Input: part model. Units: mm. Frame: model coordinates. A direction names the side the tool comes from. Coordinates: 2 decimals unless noted, no trailing zeros. Loops run counter-clockwise (first coordinate to the right, second up) from the corner with the lowest first, then second, coordinate; pieces in that order, holes last.
```python
from build123d import *

# Parameters (mm, degrees)
F2_R     = 3.75
F3_DEPTH = 33


with BuildPart() as f1:
    # F0 (on Right) → F1 (revolve)
    with BuildSketch(Plane.YZ):
        with BuildLine():
            Line((38, 45), (8, 45))
            Line((8, 45), (8, 39))
            Line((8, 39), (0, 39))
            Line((0, 39), (0, 31))
            Line((0, 31), (30, 29))
            Line((30, 29), (30, 26))
            Line((30, 26), (72, 26))
            Line((72, 26), (72, 0))
            Line((72, 0), (90, 0))
            Line((90, 0), (90, 32))
            Line((90, 32), (93, 32))
            Line((93, 32), (93, 39))
            Line((93, 39), (60, 39))
            Line((60, 39), (45.8678821818, 29.1045845728))
            ThreePointArc((45.8678821818, 29.1045845728), (40.6912569338, 28.7652906284), (38, 33.2003447942))
            Line((38, 33.2003447942), (38, 45))
        make_face()
    revolve(axis=Axis((0, 81, 0), (0, -1, 0)))

    # F2 (on face) → F3 (join)
    with BuildSketch(Plane(origin=(0, 93, 0), x_dir=(-1, 0, 0), z_dir=(0, 1, 0))):
        with BuildLine():
            Line((-8.2742985586, 74.4249113641), (-34.130188626, 18.8714128871))
            ThreePointArc((-34.130188626, 18.8714128871), (1.513291562, 38.9706293078), (35.4908216229, 16.1679182498))
            Line((35.4908216229, 16.1679182498), (8.9837408504, 74.3546347403))
            ThreePointArc((8.9837408504, 74.3546347403), (0.3772254297, 79.9162169156), (-8.2742985586, 74.4249113641))
        make_face()
        with Locations((0.3385407115, 70.4162956794)):
            Circle(F2_R, mode=Mode.SUBTRACT)
        with BuildLine():
            Line((-35.0538594373, -17.094646488), (-8.4168125088, -71.7159163408))
            ThreePointArc((-8.4168125088, -71.7159163408), (0.1390979946, -77.0518203061), (8.6756874862, -71.6850600617))
            Line((8.6756874862, -71.6850600617), (35.1153510684, -16.9679733422))
            ThreePointArc((35.1153510684, -16.9679733422), (0.0704047345, -38.9999364509), (-35.0538594373, -17.094646488))
        make_face()
        with Locations((0.1219481234, -67.551835786)):
            Circle(F2_R, mode=Mode.SUBTRACT)
    extrude(amount=-F3_DEPTH)


solid = f1.part
```
Item 1: Line query: L1, parallel to Z at x = 0, y = 91.3; L2, parallel to X at y = 61, z = 0; L3, parallel to Y at x = -38.5, z = -14. Output: solid intervals per line, ascending.
Result:
L1: z = -77.05 to -71.3, -63.8 to -32, 32 to 66.68, 74.15 to 79.91
L2: x = -39 to -26, 26 to 39
L3: y = 8 to 38
Item 2: Reachability of faces 4 (the face through (21.02, 76.73, 47.04)), 5 (the face through (-37, 8, -14)), 6 (the face through (21.922, 76.731, -44.023)), 7 (the face through (-22.4, 76.7, 44.9)), 8 (the face through (30, 38, 17)) from +Z, -Z, +X, -X, +Y, -Y: full face, straight path, thin tool, end or side. Return the list, or none.
Result:
face 4: +Z, +X, +Y
face 5: -Y
face 6: -Z, +X, +Y
face 7: +Z, -X, +Y
face 8: none
Item 3: Section query A-A (y = 78). Output: boundary loops of the cut face in (x, z), then the cut area to 3 significant figures.
Result:
outline: (-35.49, 16.17) arc R39 ccw to (-35.12, -16.97) - (-8.68, -71.69) arc R9.5 ccw to (8.42, -71.72) - (35.05, -17.09) arc R39 ccw to (34.13, 18.87) - (8.27, 74.42) arc R9.5 ccw to (-8.98, 74.35) - close; hole circle Ø7.5 at (-0.34, 70.42); hole circle Ø7.5 at (-0.12, -67.55)
area: 7,510 mm2
Item 4: Section query D-D (y = 16). Output: boundary loops of the cut face in (x, z).
Result:
outline: circle Ø90 at (0, 0); hole circle Ø59.87 at (0, 0)
Item 5: Section query B-B (x = 0). Count the separate pieces of the cut face and the enclosed holes in it, then the cut area to 3 significant figures.
Result:
separate pieces: 3
enclosed holes: 0
area: 5,250 mm2
Item 6: Section query C-C (z = 0). Output: boundary loops of the cut face in (x, y), then the cut area to 3 significant figures.
Result:
outline: (-45, 8) - (-39, 8) - (-39, 0) - (-31, 0) - (-29, 30) - (-26, 30) - (-26, 72) - (26, 72) - (26, 30) - (29, 30) - (31, 0) - (39, 0) - (39, 8) - (45, 8) - (45, 38) - (33.2, 38) arc R5 cw to (29.1, 45.87) - (39, 60) - (39, 93) - (32, 93) - (32, 90) - (-32, 90) - (-32, 93) - (-39, 93) - (-39, 60) - (-29.1, 45.87) arc R5 cw to (-33.2, 38) - (-45, 38) - close
area: 3,140 mm2
Item 7: Contact query for flat-ended pins moving along their axis: P1, Ø8.5, axis at x = -0.34, z = 70.42, coming from the -Y side; P2, Ø19, axis at x = 9, z = 8, coming from the +Y side; P3, Ø4, axis at x = 7.5, z = -35, coming from the -Y side; P4, Ø10, axis at y = 27.5, z = 14.5, coming from the -X side. Output: stop coordinate, or through.
Result:
P1: stops at y = 60
P2: stops at y = 90
P3: stops at y = 0
P4: stops at x = -43.99
Item 8: Mould query, pull axis X, two halves, no side actions, for faces 1 (the face through (-1.301, 46.554, -29.556)), 2 (the face through (-1, 60, 51)), 3 (the face through (0.366, 76.731, -63.834)). Classes: +X half, -X half, draft (parallel to the pull), parting line (faces both ways), or undercut.
Result:
face 1: parting line
face 2: draft
face 3: undercut
